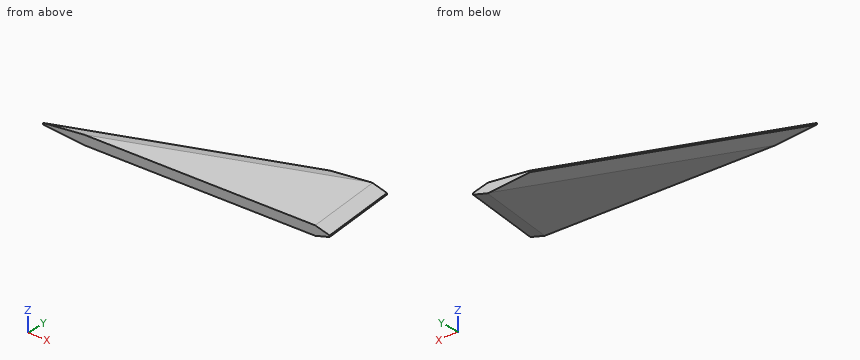
from build123d import *
from OCP.BRepFilletAPI import BRepFilletAPI_MakeChamfer

# Parameters (mm, degrees)
BOSS_EXTRUDE1_DEPTH = 1.2192
CHAMFER1_SIZE       = 3.81
CHAMFER1_SIZE2      = 1.0287
CHAMFER2_SIZE       = 3.81
CHAMFER2_SIZE2      = 1.0287


with BuildPart() as part:
    # Sketch1 → Boss-Extrude1 (new, symmetric)
    with BuildSketch(Plane.XY):
        Polygon((0, 0), (58.42, 21.59), (73.66, 21.59), (76.2, 0), align=None)
    extrude(amount=BOSS_EXTRUDE1_DEPTH, both=True)

    # Chamfer1: one chamfer whose edges measure the first distance from different faces: ONE call of the kernel's chamfer builder (chamfer() names one face for all edges)
    chamfer1_edges_1 = [part.edges().sort_by_distance(p)[0] for p in [
        (29.21, 10.795, 1.2192),
    ]]
    chamfer1_side_1 = [part.faces().sort_by_distance(p)[0] for p in [
        (48.965555556, 8.396111111, 1.2192),
    ]]
    chamfer1_edges_2 = [part.edges().sort_by_distance(p)[0] for p in [
        (29.21, 10.795, -1.2192),
    ]]
    chamfer1_side_2 = [part.faces().sort_by_distance(p)[0] for p in [
        (48.965555556, 8.396111111, -1.2192),
    ]]
    chamfer1 = BRepFilletAPI_MakeChamfer(part.part.solid().wrapped)
    for e in chamfer1_edges_1:
        chamfer1.Add(CHAMFER1_SIZE, CHAMFER1_SIZE2, e.wrapped, chamfer1_side_1[0].wrapped)  # the first distance lies on this face
    for e in chamfer1_edges_2:
        chamfer1.Add(CHAMFER1_SIZE, CHAMFER1_SIZE2, e.wrapped, chamfer1_side_2[0].wrapped)  # the first distance lies on this face
    add(Compound.cast(chamfer1.Shape()), mode=Mode.REPLACE)

    # Chamfer2: one chamfer whose edges measure the first distance from different faces: ONE call of the kernel's chamfer builder (chamfer() names one face for all edges)
    chamfer2_edges_1 = [part.edges().sort_by_distance(p)[0] for p in [
        (74.93, 10.795, -1.2192),
    ]]
    chamfer2_side_1 = [part.faces().sort_by_distance(p)[0] for p in [
        (53.47852905, 7.636921414, -1.2192),
    ]]
    chamfer2_edges_2 = [part.edges().sort_by_distance(p)[0] for p in [
        (74.93, 10.795, 1.2192),
    ]]
    chamfer2_side_2 = [part.faces().sort_by_distance(p)[0] for p in [
        (53.47852905, 7.636921414, 1.2192),
    ]]
    chamfer2 = BRepFilletAPI_MakeChamfer(part.part.solid().wrapped)
    for e in chamfer2_edges_1:
        chamfer2.Add(CHAMFER2_SIZE, CHAMFER2_SIZE2, e.wrapped, chamfer2_side_1[0].wrapped)  # the first distance lies on this face
    for e in chamfer2_edges_2:
        chamfer2.Add(CHAMFER2_SIZE, CHAMFER2_SIZE2, e.wrapped, chamfer2_side_2[0].wrapped)  # the first distance lies on this face
    add(Compound.cast(chamfer2.Shape()), mode=Mode.REPLACE)


solid = part.part
CAD build for the part. Positions are in the model's coordinates, mm. Round coordinates to 2 decimals unless told otherwise and drop trailing zeros. Loops run counter-clockwise (first coordinate to the right, second up) from the corner with the lowest first, then second, coordinate; pieces in that order, holes last.
(1) Cut at A-A (y = 9). Give the cut face in (x, z).
(2) Drop a flat-ended pin along its axis: pin 1 (1 mm diameter, centred on x = 48, y = 16, fed in from -Z). Give the stop position or say it passes through.
(3) Cut at D-D (x = 44). Give the cut face in (y, z), plus the area to 3 significant figures.
(4) Cut at B-B (x = 22). Give the cut face in (y, z), plus the area to 3 significant figures.
(5) Cut at C-C (z = 0.65). Give the cut face in (x, y), plus the area to 3 significant figures.
(6) Wall check: line 1 along Z through (x, y) = (26.5, 9); line 2 along Z through (x, y) = (48, 14); line 3 along Y through (x, z) = (56.5, 0.1). Give the ranges that are in metal, low to high.
Findings below:
1. outline: (24.35, -0.19) - (35.34, -1.22) - (71.3, -1.22) - (75.14, -0.19) - (75.14, 0.19) - (71.3, 1.22) - (35.34, 1.22) - (24.35, 0.19) - close
2. pin 1: stops at z = -0.77
3. outline: (0, -1.22) - (12.2, -1.22) - (16.26, -0.19) - (16.26, 0.19) - (12.2, 1.22) - (0, 1.22) - close
3. area: 35.5 mm2
4. outline: (0, -1.22) - (4.07, -1.22) - (8.13, -0.19) - (8.13, 0.19) - (4.07, 1.22) - (0, 1.22) - close
4. area: 15.6 mm2
5. outline: (4.91, 0) - (74.49, 0) - (71.95, 21.59) - (63.33, 21.59) - close
5. area: 844 mm2
6. line 1: z = -0.39 to 0.39
6. line 2: z = -1.14 to 1.14
6. line 3: y = 0 to 20.88
